Verification items for the finished model (mm, model axes). Face numbers are marked on the shaded views. Round coordinates to 2 decimals unless told otherwise and drop trailing zeros. Write each loop counter-clockwise with the first axis right and the second up, starting at its lowest first coordinate (ties: lowest second). Pieces come first, ordered by that corner, then holes. Notation, with made-up numbers: (82.5, 42) - (122.5, 42) arc R30 ccw to (122.5, 78) - close; hole circle Ø4 at (60, -31). An arc over 180 degrees is marked (long way). Write each question's results on one line, items separated by ' | '.
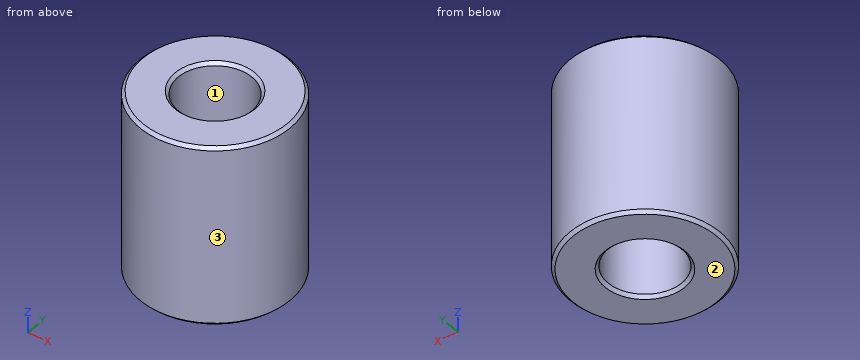
Autodesk Inventor part; units mm, degrees
ref_plane "YZ Plane" through (0, 0, 0) normal (1, 0, 0) x (0, 1, 0)
ref_plane "XZ Plane" through (0, 0, 0) normal (0, 1, 0) x (-1, 0, 0)
ref_plane "XY Plane" through (0, 0, 0) normal (0, 0, 1) x (1, 0, 0)
sketch "スケッチ1" plane through (0, 0, 0) normal (0, 0, 1) x (1, 0, 0)
  circle A0 centre (0, 0) radius 2.5
  dimension "d0" = 5
extrude "押し出し1" add sketch "スケッチ1" along normal blind 6
sketch "スケッチ2" plane through (0, 0, 6) normal (0, 0, 1) x (1, 0, 0)
  circle A0 centre (0, 0) radius 2.5 construction
hole "穴1" at (0, 0, 6) direction (0, 0, -1) diameter 2.459 end through all
chamfer "面取り1" distance 0.1 angle 45 4 edges at (0, 1.2295, 6) (-2.5, 0, 6) (-2.5, 0, 0) (0, 1.2295, 0)
properties part number "SB-305060" material "真鍮、ソフト イエロー"
(1) Thickness scan on L1, parallel to Y at x = 0, z = 2; L2, parallel to Y at x = -1.05, z = 5.7; L3, parallel to X at y = 0.55, z = 2.8. Record the ranges inside material, lowest first.
Answer:
L1: -2.5 to -1.23, 1.23 to 2.5 | L2: -2.27 to -0.64, 0.64 to 2.27 | L3: -2.44 to -1.1, 1.1 to 2.44
(2) Section check B-B (z = 5.1). Record the cut outline in (x, y), plus the area to 3 significant figures.
Answer:
outline: circle Ø5 at (0, 0); hole circle Ø2.46 at (0, 0) | area: 14.9 mm2
(3) Mould release check, pull along X, two halves, no side actions. Record for the marked faces 1, 2 and 3: released by +X, released by -X, zero draft, split by the parting line, or undercut.
Answer:
face 1: undercut | face 2: zero draft | face 3: split by the parting line
(4) Section check A-A (y = 0). Record the cut outline in (x, z).
Answer:
outline: (-2.5, 0.1) - (-2.4, 0) - (-1.33, 0) - (-1.23, 0.1) - (-1.23, 5.9) - (-1.33, 6) - (-2.4, 6) - (-2.5, 5.9) - close; (1.23, 0.1) - (1.33, 0) - (2.4, 0) - (2.5, 0.1) - (2.5, 5.9) - (2.4, 6) - (1.33, 6) - (1.23, 5.9) - close
(5) Go/stop test with a flat-tipped pin: pin 1 Ø2 at (x, y) = (0, 0) entering from +Z. Record where the tip stops, or that it passes through.
Answer:
pin 1: through
